Check sheet for the modelled part. Datum: model origin and axes. Units: mm. Round coordinates to 2 decimals unless told otherwise and drop trailing zeros. Loops run counter-clockwise (first coordinate to the right, second up) from the corner with the lowest first, then second, coordinate; pieces in that order, holes last. Notation, with made-up numbers: (44, 54) - (81, 54) arc R18 ccw to (81, 78) - close; hole circle Ø7 at (-38.5, -14.75). An arc over 180 degrees is marked (long way). Answer in a Markdown table with one row per item. Add a question column.
(1) Gauge pin test, flat ends, axial feed: pin 1 (1 mm diameter, centred on y = 7307, z = 279.5, fed in from +X); pin 2 (6 mm diameter, centred on y = 7643, z = 355, fed in from -X); pin 3 (1.5 mm diameter, centred on y = 7334, z = 531.5, fed in from +X). Record the tip position at first contact, or that the pin passes through.
(2) Cross-section at B-B on x = -8000.5. Enter the section's corners in (y, z).
(3) Cross-section at C-C on y = 7234.5. Enter the section's corners in (x, z), then the cut area to 3 significant figures.
(4) Thickness scan on line 1 along Y through (x, z) = (-8091, 165); line 2 along Y through (x, z) = (-8123, 398.5); line 3 along X through (y, z) = (7297, 526). Record the ranges inside material, lowest first.
(5) Cross-section at A-A on z = 520. Enter the section's corners in (x, y), then the cut area to 3 significant figures.
from build123d import *

# Parameters (mm, degrees)
EXTRUDE_1_DEPTH = 480
SCALE_1_SCALE   = 1.3


with BuildPart() as part:
    # 草图1 → 凸台-拉伸1 (new body)
    with BuildSketch(Plane.XY):
        with BuildLine():
            Line((-6833.3126292, 5666.028511287), (-6759.14855055, 5437.774947376))
            ThreePointArc((-6759.14855055, 5437.774947376), (-6502.809901268, 5499.3164122), (-6240, 5520))
            Line((-6240, 5520), (-6240, 5760))
            ThreePointArc((-6240, 5760), (-6540.354172877, 5736.361613943), (-6833.3126292, 5666.028511287))
        make_face()
        with BuildLine():
            ThreePointArc((-6240, 5520), (-5977.190098732, 5499.3164122), (-5720.85144945, 5437.774947376))
            Line((-5720.85144945, 5437.774947376), (-5683.769410125, 5551.901729331))
            Line((-5683.769410125, 5551.901729331), (-5646.6873708, 5666.028511287))
            ThreePointArc((-5646.6873708, 5666.028511287), (-5939.645827123, 5736.361613943), (-6240, 5760))
            Line((-6240, 5760), (-6240, 5520))
        make_face()
        with BuildLine():
            ThreePointArc((-6240, 5760), (-5939.645827123, 5736.361613943), (-5646.6873708, 5666.028511287))
            Line((-5646.6873708, 5666.028511287), (-5551.170243986, 5960))
            Line((-5551.170243986, 5960), (-6928.829756014, 5960))
            Line((-6928.829756014, 5960), (-6833.3126292, 5666.028511287))
            ThreePointArc((-6833.3126292, 5666.028511287), (-6540.354172877, 5736.361613943), (-6240, 5760))
        make_face()
    extrude(amount=EXTRUDE_1_DEPTH)


with BuildPart() as part_1:
    # 缩放比例1: scaled about (0, 0, 0)
    add(part.part.scale(SCALE_1_SCALE))


solid = part_1.part
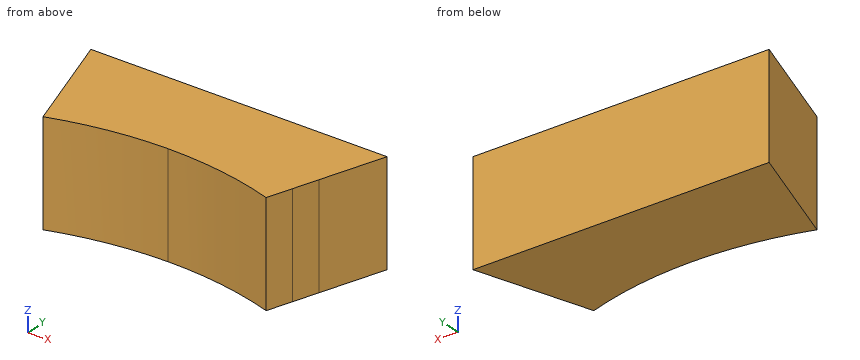
Answers:
| question | item | result |
|---|---|---|
| 1 | pin 1 | stops at x = -7359.65 |
| 1 | pin 2 | stops at x = -8974.34 |
| 1 | pin 3 | stops at x = -7350.79 |
| 2 | outline | (7173.15, 0) - (7748, 0) - (7748, 624) - (7173.15, 624) - close |
| 3 | outline | (-8840.63, 0) - (-7383.37, 0) - (-7383.37, 624) - (-8840.63, 624) - close |
| 3 | area | 909,000 mm^2 |
| 4 | line 1 | y = 7175.9 to 7748 |
| 4 | line 2 | y = 7175.97 to 7748 |
| 4 | line 3 | x = -8860.94 to -7363.06 |
| 5 | outline | (-9007.48, 7748) - (-8786.89, 7069.11) arc R2184 cw to (-7437.11, 7069.11) - (-7216.52, 7748) - close |
| 5 | area | 969,000 mm^2 |
